Geometry: final body of the model. Coordinates: model frame, mm. Coordinates: 2 decimals unless noted, no trailing zeros. Write each loop counter-clockwise with the first axis right and the second up, starting at its lowest first coordinate (ties: lowest second). Pieces come first, ordered by that corner, then holes.
from build123d import *

# Parameters (mm, degrees)
SKETCH_1_R               = 59.5
SKETCH_1_R_2             = 52.5
EXTRUDE_1_DEPTH          = 25
SKETCH_2_R               = 1.55
CUT_EXTRUDE_1_DEPTH      = 88.780977438
PATTERN_CIRCULAR_1_COUNT = 18


with BuildPart() as part:
    # 草图1 → 凸台-拉伸1 (new body)
    with BuildSketch(Plane(origin=(0, 0, 0), x_dir=(0, 0, -1), z_dir=(1, 0, 0))):
        Circle(SKETCH_1_R)
        Circle(SKETCH_1_R_2, mode=Mode.SUBTRACT)
    extrude(amount=EXTRUDE_1_DEPTH)

    # 草图2 → 切除-拉伸1 (cut, through all)
    with BuildSketch(Plane(origin=(25, 0, 0), x_dir=(0, 0, -1), z_dir=(1, 0, 0))):
        with Locations((0, 55.5)):
            Circle(SKETCH_2_R)
    cut_extrude_1 = extrude(amount=-CUT_EXTRUDE_1_DEPTH, mode=Mode.SUBTRACT)

    # 阵列(圆周)1: 切除-拉伸1 ×18 about axis
    pattern_circular_1_axis = Axis((0, 0, 0), (1, 0, 0))
    for i in range(1, PATTERN_CIRCULAR_1_COUNT):
        add(cut_extrude_1.rotate(pattern_circular_1_axis, i * 360 / PATTERN_CIRCULAR_1_COUNT), mode=Mode.SUBTRACT)


solid = part.part
Item 1: Material intervals for probe 1 along Y at (x, z) = (7, 0); probe 2 along Z at (x, y) = (9.5, -9); probe 3 along Y at (x, z) = (9, 53.5), sorted ascending.
Derived:
probe 1: y = -59.5 to -57.05, -53.95 to -52.5, 52.5 to 53.95, 57.05 to 59.5
probe 2: z = -58.82 to -56.07, -53.24 to -51.72, 51.72 to 53.24, 56.07 to 58.82
probe 3: y = -26.04 to -10.67, -8.61 to 8.61, 10.67 to 26.04
Item 2: Section D-D, the plane y = 55.5. Output: boundary loops of the cut face in (x, z).
Derived:
outline: (0, -21.45) - (25, -21.45) - (25, -1.55) - (0, -1.55) - close; (0, 1.55) - (25, 1.55) - (25, 21.45) - (0, 21.45) - close
Item 3: Pull-direction query (Z, two-part tool) for faces 1 (the cylindrical face through (12.32, 50.17, -31.99)), 2 (the cylindrical face through (12.675, -10.685, 53.514)), 3 (the cylindrical face through (12.675, 57.037, 0.202)), 4 (the flat face through (25, 0, -53)); classes: released by +Z, released by -Z, zero draft, split by the parting line, or undercut.
Derived:
face 1: split by the parting line
face 2: undercut
face 3: undercut
face 4: zero draft
Item 4: Pin query (flat end, axial travel): pin 1 (8 mm diameter, centred on x = 20.5, y = -19.5, fed in from -Z); pin 2 (4 mm diameter, centred on y = -27.75, z = -48.06, fed in from -X); pin 3 (6 mm diameter, centred on x = 5, y = -20.5, fed in from +Z); pin 4 (3 mm diameter, centred on x = 20.5, z = 14, fed in from -Y). Return the tip coordinate at first contact, or that it passes through.
Derived:
pin 1: stops at z = -57.45
pin 2: stops at x = 0
pin 3: stops at z = 56.87
pin 4: stops at y = -58.17
Item 5: Section A-A, the plane z = 0. Output: boundary loops of the cut face in (x, y).
Derived:
outline: (0, -59.5) - (25, -59.5) - (25, -57.05) - (0, -57.05) - close; (0, -53.95) - (25, -53.95) - (25, -52.5) - (0, -52.5) - close; (0, 52.5) - (25, 52.5) - (25, 53.95) - (0, 53.95) - close; (0, 57.05) - (25, 57.05) - (25, 59.5) - (0, 59.5) - close
Item 6: Section C-C, the plane x = 15. State how many separate pieces and enclosed holes the cut face has, plus the area to 3 significant figures.
Derived:
separate pieces: 1
enclosed holes: 19
area: 2,330 mm2
Item 7: Section B-B, the plane y = 0. Output: boundary loops of the cut face in (x, z).
Derived:
outline: (0, -59.5) - (25, -59.5) - (25, -52.5) - (0, -52.5) - close; (0, 52.5) - (25, 52.5) - (25, 59.5) - (0, 59.5) - close
